Input: part model. Units: mm. Frame: model coordinates. A direction names the side the tool comes from. Round coordinates to 2 decimals unless told otherwise and drop trailing zeros. Loops run counter-clockwise (first coordinate to the right, second up) from the corner with the lowest first, then second, coordinate; pieces in that order, holes last.
1) Section A-A, the plane x = -12. Return loops of the section in (y, z).
2) Section D-D, the plane x = 0. Return loops of the section in (y, z).
3) Draft query along X for faces 1 (the face through (0, -5, 2)), 2 (the face through (-5, 15, 2)), 3 (the face through (-19.48, 28.76, 1.97)), 4 (the face through (7, 0, 2)). Return one class per face: pulls with the +X half, pulls with the -X half, needs draft (parallel to the pull), parting line crosses it, or undercut.
4) Ray query, line 1 along Y through (x, z) = (-12.5, 0.65); line 2 along X through (y, z) = (21, 0.35); line 3 along X through (y, z) = (-2, 3). Return the intervals inside material, ascending.
5) Access query for faces 5 (the face through (0, -9, 2)), 6 (the face through (-9, 15, 2)), 7 (the face through (-10, 29, 2)), 8 (the face through (-19, 2, 2)), 9 (the face through (-18.708, 31.478, 1.972)). Directions: +Z, -Z, +X, -X, +Y, -Y. A direction counts if a zero-diameter tool reaches every point of the face in a straight line with its end or side. Return the directions, or none.
6) Section C-C, the plane z = 3.35. Return loops of the section in (x, y).
7) Section B-B, the plane y = -3.5. Return loops of the section in (x, z), and give its area (3 significant figures).
8) First-contact query: pin 1 (1.2 mm diameter, centred on y = 1, z = 3, fed in from -X); pin 2 (2 mm diameter, centred on x = 6.5, z = 2.5, fed in from +Y); pin 3 (2 mm diameter, centred on x = -12.5, z = 2.5, fed in from -Y). Flat tips, straight axial feed; report the tip coordinate or a pass-through.
from build123d import *

# Parameters (mm, degrees)
PAD_DEPTH = 4


with BuildPart() as part:
    # Sketch → Pad (new body)
    with BuildSketch(Plane.XY):
        with BuildLine():
            Line((-5, 29), (-5, 0))
            ThreePointArc((-5, 0), (0, -5), (5, 0))
            Line((5, 0), (9, 0))
            ThreePointArc((-9, 0), (0, -9), (9, 0))
            Line((-19, 0), (-9, 0))
            Line((-19, 4), (-19, 0))
            Line((-9, 4), (-19, 4))
            Line((-9, 25), (-9, 4))
            Line((-15, 25), (-9, 25))
            ThreePointArc((-18.46412, 26.999997), (-17.00001, 25.535892), (-15, 25))
            Line((-20.464122, 30.464102), (-18.46412, 26.999997))
            Line((-17.00002, 32.464102), (-20.464122, 30.464102))
            Line((-15.00002, 29), (-17.00002, 32.464102))
            Line((-5, 29), (-15.00002, 29))
        make_face()
    extrude(amount=PAD_DEPTH)


solid = part.part
Final values:
1. outline: (0, 0) - (4, 0) - (4, 4) - (0, 4) - close; (25, 0) - (29, 0) - (29, 4) - (25, 4) - close
2. outline: (-9, 0) - (-5, 0) - (-5, 4) - (-9, 4) - close
3. face 1: undercut
3. face 2: pulls with the +X half
3. face 3: pulls with the -X half
3. face 4: needs draft
4. line 1: y = 0 to 4, 25 to 29
4. line 2: x = -9 to -5
4. line 3: x = -8.77 to -4.58, 4.58 to 8.77
5. face 5: +Z, -Z, -Y
5. face 6: +Z, -Z, -X
5. face 7: +Z, -Z, +X, +Y
5. face 8: +Z, -Z, -X, -Y
5. face 9: +Z, -Z, -X, +Y
6. outline: (-20.46, 30.46) - (-18.46, 27) arc R4 ccw to (-15, 25) - (-9, 25) - (-9, 4) - (-19, 4) - (-19, 0) - (-9, 0) arc R9 ccw to (9, 0) - (5, 0) arc R5 cw to (-5, 0) - (-5, 29) - (-15, 29) - (-17, 32.46) - close
7. outline: (-8.29, 0) - (-3.57, 0) - (-3.57, 4) - (-8.29, 4) - close; (3.57, 0) - (8.29, 0) - (8.29, 4) - (3.57, 4) - close
7. area: 37.8 mm2
8. pin 1: stops at x = -19
8. pin 2: stops at y = 0
8. pin 3: stops at y = 0
